Study the drawing (mm; zero at the part's minimum x, y, z) and answer. Round coordinates to 2 decimals unless told otherwise and drop trailing zeros. Order: outer loops, then holes, each group sorted by start corner. A loop starts at its lowest first (then second) coordinate and runs counter-clockwise, first axis right, second up. Notation, with made-up numbers: (63.5, 14) - (86.5, 14) arc R10 ccw to (86.5, 30) - close; hole circle Ø3 at (85, 31.5). An arc over 180 degrees is marked (long way). Use one line per item in the form item = value. Start each with the question number.
Q1. The part is cut by section A-A on y = 6. Determine the outline of the cut face in (x, z), plus the area to 3 significant figures.
Q2. Given P1, Ø1.8, axis at x = 5, y = 7, coming from the +Z side; P2, Ø1, axis at y = 4.5, z = 32.5, coming from the +X side; P3, Ø1.8, axis at x = 5, y = 5, coming from the -Z side, each flat-ended and moving along its own axis, determine where each tip first touches the part or whether it passes through.
Q3. The part is cut by section C-C on z = 18.5. Determine the outline of the cut face in (x, y), plus the area to 3 significant figures.
Q4. Find the intervals of material crossed by line 1 (Y direction, x = 6, z = 60.75); line 2 (Z direction, x = 8.75, y = 6.75); line 3 (X direction, y = 7, z = 4), in increasing order. Write a range as [from, to].
Q5. The part is cut by section D-D on y = 10.5. Determine the outline of the cut face in (x, z).
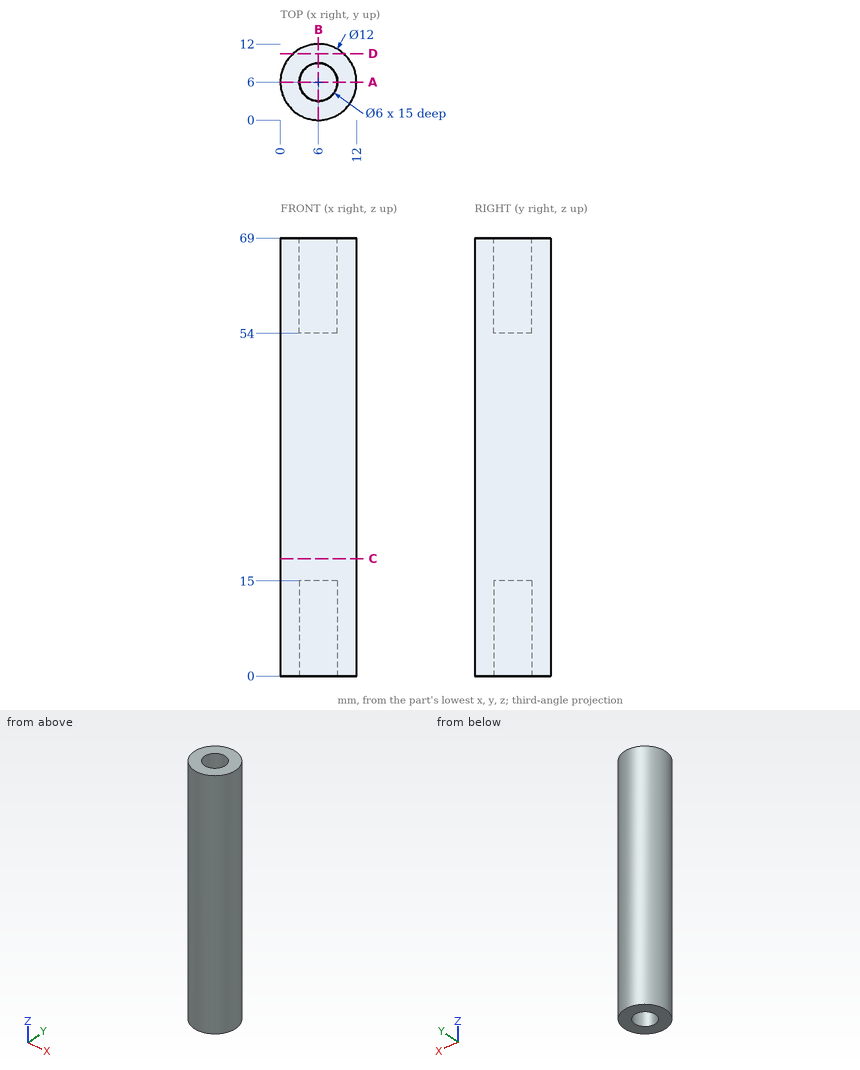
Found:
q1.outline = (0, 0) - (3, 0) - (3, 15) - (9, 15) - (9, 0) - (12, 0) - (12, 69) - (9, 69) - (9, 54) - (3, 54) - (3, 69) - (0, 69) - close
q1.area = 648 mm²
q2.P1 = 54
q2.P2 = 11.92
q2.P3 = 15
q3.outline = circle Ø12 at (6, 6)
q3.area = 113 mm²
q4.line_1 = [0, 3], [9, 12]
q4.line_2 = [15, 54]
q4.line_3 = [0.08, 3.17], [8.83, 11.92]
q5.outline = (2.03, 0) - (9.97, 0) - (9.97, 69) - (2.03, 69) - close
